```python
from build123d import *

# Parameters (mm, degrees)
CUT_EXTRUDE_1_DEPTH      = 10
PATTERN_CIRCULAR_1_COUNT = 3
FILLET_1_R               = 0.5


with BuildPart() as part:
    # Эскиз1 → Повернуть1 (revolve)
    with BuildSketch(Plane(origin=(0, 0, 0), x_dir=(0, 0, -1), z_dir=(1, 0, 0)), mode=Mode.PRIVATE) as revolve_1_sk:
        Polygon((-9, 0), (-9, 2), (1, 2), (1, 5), (3, 5), (3.7, 5.5), (8.916460066, 17.5), (23.4, 17.5), (23.4, 16), (9.9, 16), (7.009211714, 9.35), (7.009211714, 5), (9, 5), (9, 0), align=None)
    revolve(revolve_1_sk.sketch.rotate(Axis((0, 0, -9), (0, 0, -1)), 90), axis=Axis((0, 0, -9), (0, 0, -1)))

    # Эскиз2 → Вырез-Вытянуть1 (cut)
    with BuildSketch(Plane.XY.offset(-1)):
        with BuildLine():
            Line((1.55, 14.5641447), (-1.55, 14.5641447))
            ThreePointArc((-1.55, 14.5641447), (-6.235, 9.8791447), (-1.55, 5.1941447))
            Line((-1.55, 5.1941447), (1.55, 5.1941447))
            ThreePointArc((1.55, 5.1941447), (6.235, 9.8791447), (1.55, 14.5641447))
        make_face()
    cut_extrude_1 = extrude(amount=-CUT_EXTRUDE_1_DEPTH, mode=Mode.SUBTRACT)

    # Круговой массив1: Вырез-Вытянуть1 ×3 about axis
    pattern_circular_1_axis = Axis((0, 0, 0), (0, 0, 1))
    for i in range(1, PATTERN_CIRCULAR_1_COUNT):
        add(cut_extrude_1.rotate(pattern_circular_1_axis, i * 360 / PATTERN_CIRCULAR_1_COUNT), mode=Mode.SUBTRACT)

    # Скругление1
    fillet_1_edges = [part.edges().sort_by_distance(p)[0] for p in [
        (-17.5, 0, -23.4),
        (-17.5, 0, -8.916460066),
        (-5, 0, -1),
    ]]
    fillet(fillet_1_edges, radius=FILLET_1_R)


solid = part.part
```
Geometry: final body of the model. Coordinates: model frame, mm. A direction names the side the tool comes from. Coordinates: 2 decimals unless noted, no trailing zeros. Loops run counter-clockwise (first coordinate to the right, second up) from the corner with the lowest first, then second, coordinate; pieces in that order, holes last. Notation, with made-up numbers: M 89.25,55.5 L 117.25,55.5 A15 ccw 117.25,80.5 Z; hole C 3.25,7 d8. An arc over 180 degrees is marked long. Put each result on its own line as item: value.
(1) Cut plane B-B on z = -17. Return the cut outline in (x, y).
Answer sheet:
outline: C 0,0 d35; hole C 0,0 d32
(2) Cut plane A-A on z = 2.5. Return the cut outline in (x, y), then the cut area to 3 significant figures.
Answer sheet:
outline: C 0,0 d4
area: 12.6 mm^2
(3) Draft query along X for faces 1 (the face through (13, 10, -23.4)), 2 (the face through (-4.487, -2.616, -5.114)), 3 (the face through (-10.64, 0.9, -6.66)). Return one class per face: pulls with the +X half, pulls with the -X half, needs draft (parallel to the pull), parting line crosses it, or undercut.
Answer sheet:
face 1: needs draft
face 2: pulls with the -X half
face 3: undercut
(4) Material intervals for probe 1 along Y at (x, z) = (0, -13); probe 2 along Z at (x, y) = (-3, 1); probe 3 along Y at (x, z) = (4, -11.5), sorted ascending.
Answer sheet:
probe 1: y = -17.5 to -16, 16 to 17.5
probe 2: z = -9 to -1
probe 3: y = -17.04 to -15.49, 15.49 to 17.04
(5) Access query for faces 4 (the face through (12.602, -7.301, -8.464)), 5 (the face through (0, 0, 9)), 6 (the face through (4.51, -2.58, -5.11)), 7 (the face through (0, 2, 4)), 8 (the face through (-2, 5, -7.009)). Directions: +Z, -Z, +X, -X, +Y, -Y. A direction counts if a zero-diameter tool reaches every point of the face in a straight line with its end or side. Return the directions, or none.
Answer sheet:
face 4: +Z, -Z
face 5: +Z, +X, -X, +Y, -Y
face 6: +Z, -Z, +X
face 7: +Z
face 8: -Z
(6) First-contact query: pin 1 (4 mm diameter, centred on y = -13, z = -17, fed in from +X); pin 2 (3 mm diameter, centred on x = 4.5, z = -5.5, fed in from -Y); pin 3 (19 mm diameter, centred on x = 0, y = 0, fed in from -Z). Flat tips, straight axial feed; report the tip coordinate or a pass-through.
Answer sheet:
pin 1: stops at x = 13.61
pin 2: stops at y = -12.33
pin 3: stops at z = -9
